```python
from build123d import *

# Parameters (mm, degrees)
BOSS_EXTRUDE1_DEPTH       = 15
BOSS_EXTRUDE5_START       = 23.320459961
BOSS_EXTRUDE5_OUTLINE_W   = 12
BOSS_EXTRUDE5_OUTLINE_H   = 10
BOSS_EXTRUDE5_DEPTH       = 6.679540039
BOSS_EXTRUDE5_START_2     = -15
BOSS_EXTRUDE5_2_DEPTH     = 12
BOSS_EXTRUDE5_3_OUTLINE_W = 2.674630913
BOSS_EXTRUDE5_3_OUTLINE_H = 10
BOSS_EXTRUDE5_3_DEPTH     = 4.684664465
CUT_EXTRUDE1_DEPTH        = 45.229515032
FILLET1_R                 = 1


with BuildPart() as part:
    # Sketch1 → Boss-Extrude1 (new, symmetric)
    with BuildSketch(Plane.XY):
        with BuildLine():
            Line((-35, 0), (-22.5, 0))
            ThreePointArc((-22.5, 0), (0, -22.5), (22.5, 0))
            Line((22.5, 0), (35, 0))
            Line((35, 0), (35, -3))
            Line((35, -3), (25.322914524, -3))
            ThreePointArc((25.322914524, -3), (0, -25.5), (-25.322914524, -3))
            Line((-25.322914524, -3), (-35, -3))
            Line((-35, -3), (-35, 0))
        make_face()
    extrude(amount=BOSS_EXTRUDE1_DEPTH, both=True)

    # Boss-Extrude5: read off the stored shape, not the designer's step
    # Boss-Extrude5 outline → Boss-Extrude5 (add)
    with BuildSketch(Plane.YZ.offset(BOSS_EXTRUDE5_START)):
        with Locations((-9, 0)):
            Rectangle(BOSS_EXTRUDE5_OUTLINE_W, BOSS_EXTRUDE5_OUTLINE_H)
    boss_extrude5 = extrude(amount=BOSS_EXTRUDE5_DEPTH)

    # Boss-Extrude5 2 outline → Boss-Extrude5 2 (add)
    with BuildSketch(Plane(origin=(0, 0, 0), x_dir=(1, 0, 0), z_dir=(0, 1, 0)).offset(BOSS_EXTRUDE5_START_2)):
        with BuildLine():
            ThreePointArc((30, -5), (35, 0), (30, 5))
            Line((30, 5), (30, -5))
        make_face()
    boss_extrude5_2 = extrude(amount=BOSS_EXTRUDE5_2_DEPTH)

    # Boss-Extrude5 3 outline → Boss-Extrude5 3 (add)
    with BuildSketch(Plane(origin=(0, 0, 0), x_dir=(1, 0, 0), z_dir=(0, 1, 0)).offset(BOSS_EXTRUDE5_START_2)):
        with Locations((21.983144505, 0)):
            Rectangle(BOSS_EXTRUDE5_3_OUTLINE_W, BOSS_EXTRUDE5_3_OUTLINE_H)
    boss_extrude5_3 = extrude(amount=BOSS_EXTRUDE5_3_DEPTH)

    # Sketch4_5 → Cut-Extrude1 (cut, symmetric)
    with BuildSketch(Plane.XZ.offset(3)):
        with BuildLine():
            ThreePointArc((33.25, 0), (32.298097039, 2.298097039), (30, 3.25))
            Line((30, 3.25), (30, -3.25))
            ThreePointArc((30, -3.25), (32.298097039, -2.298097039), (33.25, 0))
        make_face()
        with BuildLine():
            Line((30, -3.25), (30, 3.25))
            ThreePointArc((30, 3.25), (26.75, 0), (30, -3.25))
        make_face()
    cut_extrude1 = extrude(amount=CUT_EXTRUDE1_DEPTH, both=True, mode=Mode.SUBTRACT)

    # Mirror1: Boss-Extrude5, Boss-Extrude5 2, Boss-Extrude5 3, Cut-Extrude1 across plane
    add(boss_extrude5.mirror(Plane(origin=(0, 0, 0), x_dir=(0, 0, 1), z_dir=(1, 0, 0))))
    add(boss_extrude5_2.mirror(Plane(origin=(0, 0, 0), x_dir=(0, 0, 1), z_dir=(1, 0, 0))))
    add(boss_extrude5_3.mirror(Plane(origin=(0, 0, 0), x_dir=(0, 0, 1), z_dir=(1, 0, 0))))
    add(cut_extrude1.mirror(Plane(origin=(0, 0, 0), x_dir=(0, 0, 1), z_dir=(1, 0, 0))), mode=Mode.SUBTRACT)

    # Fillet1
    fillet1_edges = [part.edges().sort_by_distance(p)[0] for p in [
        (-30.161457262, -3, -15),
        (-35, -1.5, -15),
        (-28.75, 0, -15),
        (0, -22.5, -15),
        (-35, -1.5, 15),
        (-30.161457262, -3, 15),
        (0, -25.5, 15),
        (30.161457262, -3, 15),
        (35, -1.5, 15),
        (28.75, 0, 15),
        (0, -22.5, 15),
        (28.75, 0, -15),
        (-28.75, 0, 15),
        (35, -1.5, -15),
        (30.161457262, -3, -15),
        (0, -25.5, -15),
    ]]
    fillet(fillet1_edges, radius=FILLET1_R)


solid = part.part
```
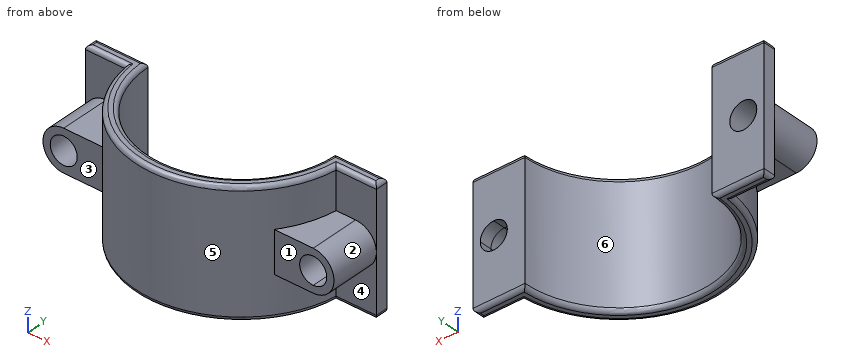
Could you check a few things on this model? Use its own coordinates, in mm. Face numbers are marked on the shaded views. A direction names the side the tool comes from. Round coordinates to 2 decimals unless told otherwise and drop trailing zeros. Write each loop counter-clockwise with the first axis right and the second up, starting at its lowest first coordinate (ties: lowest second). Pieces come first, ordered by that corner, then holes. Notation, with made-up numbers: M -4.75,62.25 L 26.25,62.25 A15 ccw 26.25,80.25 Z; hole C 88,50 d10. An arc over 180 degrees is marked long. Answer in a Markdown table with one row per item. Add a question column.
Q1. Will these pins go through, and if not, where does the flat tip stop? pin 1 Ø8.5 at (x, z) = (-30, 0) entering from -Y; pin 2 Ø7.5 at (x, z) = (-31.5, 9) entering from -Y; pin 3 Ø8 at (y, z) = (-15.5, -5) entering from -X.
Q2. If we mould it in two halves opening along X, with no side actions, what happens to the marked faces 4, 5 and 6? For each: +X half, -X half, draft (parallel to the pull), parting line (faces both ways), or undercut.
Q3. Imagine slicing it at B-B (x = 0). Please give me the cut outline in (y, z).
Q4. On a 3-axis mill with a long thin cutter (end or side, diameter ignored), from which of +Z, -Z, +X, -X, +Y, -Y can I reach the whole of each face in a straight line? I mean the marked faces 1, 2 and 3. Say none if no direction works.
Q5. Imagine slicing it at C-C (z = -7). Please give me the cut outline in (x, y), then the cut area to 3 significant figures.
Q6. If I drill on line 1 (Z direction, x = -30, y = -3.5); line 2 (X direction, y = -11, z = 0); line 3 (X direction, y = -9, z = 0), over which ranges is the centre line in solid material (lowest first)? Write a range as from..to.
Values:
| question | item | result |
|---|---|---|
| 1 | pin 1 | y = -15 |
| 1 | pin 2 | y = -3 |
| 1 | pin 3 | x = -34.89 |
| 2 | face 4 | draft |
| 2 | face 5 | parting line |
| 2 | face 6 | undercut |
| 3 | outline | M -25.5,-14 A1 ccw -24.5,-15 L -23.5,-15 A1 ccw -22.5,-14 L -22.5,14 A1 ccw -23.5,15 L -24.5,15 A1 ccw -25.5,14 Z |
| 4 | face 1 | +Z, -Z, +X, -Y |
| 4 | face 2 | +X, -Y |
| 4 | face 3 | +Z, -Z, -X, -Y |
| 5 | outline | M -35,-3 L -25.32,-3 A25.5 ccw 25.32,-3 L 35,-3 L 35,0 L 22.5,0 A22.5 cw -22.5,0 L -35,0 Z |
| 5 | area | 284 mm^2 |
| 6 | line 1 | -5..-3.25, 3.25..5 |
| 6 | line 2 | -35..-33.25, -26.75..-19.63, 19.63..26.75, 33.25..35 |
| 6 | line 3 | -35..-33.25, -26.75..-20.62, 20.62..26.75, 33.25..35 |
